from build123d import *

# Parameters (mm, degrees)
CROQUIS1_R              = 23.05
SALIENTE_EXTRUIR1_DEPTH = 25
CROQUIS2_R              = 19.05
CORTAR_EXTRUIR1_DEPTH   = 29
CROQUIS3_R              = 23.05
CROQUIS3_R_2            = 20.5
CORTAR_EXTRUIR2_DEPTH   = 5
CROQUIS4_R              = 30
SALIENTE_EXTRUIR3_DEPTH = 20
CROQUIS5_R              = 19.05
CORTAR_EXTRUIR3_DEPTH   = 20


with BuildPart() as part:
    # Croquis1 → Saliente-Extruir1 (new body)
    with BuildSketch(Plane.XY):
        Circle(CROQUIS1_R)
    extrude(amount=SALIENTE_EXTRUIR1_DEPTH)

    # Croquis2 → Cortar-Extruir1 (cut)
    with BuildSketch(Plane(origin=(0, 0, 0), x_dir=(-1, 0, 0), z_dir=(0, 0, -1))):
        Circle(CROQUIS2_R)
    extrude(amount=-CORTAR_EXTRUIR1_DEPTH, mode=Mode.SUBTRACT)

    # Croquis3 → Cortar-Extruir2 (cut)
    with BuildSketch(Plane(origin=(0, 0, 0), x_dir=(-1, 0, 0), z_dir=(0, 0, -1))):
        Circle(CROQUIS3_R)
        Circle(CROQUIS3_R_2, mode=Mode.SUBTRACT)
    extrude(amount=-CORTAR_EXTRUIR2_DEPTH, mode=Mode.SUBTRACT)

    # Croquis4 → Saliente-Extruir3 (add)
    with BuildSketch(Plane.XY.offset(25)):
        Circle(CROQUIS4_R)
    extrude(amount=-SALIENTE_EXTRUIR3_DEPTH)

    # Croquis5 → Cortar-Extruir3 (cut)
    with BuildSketch(Plane(origin=(0, 0, 5), x_dir=(-1, 0, 0), z_dir=(0, 0, -1))):
        Circle(CROQUIS5_R)
    extrude(amount=-CORTAR_EXTRUIR3_DEPTH, mode=Mode.SUBTRACT)


solid = part.part
Geometry check sheet. Reference: the model listing, model coordinates, mm. A direction names the side the tool comes from. Round coordinates to 2 decimals unless told otherwise and drop trailing zeros. Loops run counter-clockwise (first coordinate to the right, second up) from the corner with the lowest first, then second, coordinate; pieces in that order, holes last.
Item 1: Cross-section at D-D on x = 24. Record the boundary of the cut face in (y, z), then the cut area to 3 significant figures.
Item 2: Cross-section at C-C on z = 19.75. Record the boundary of the cut face in (x, y).
Item 3: Mould release check, pull along Y, two halves, no side actions. Record for faces 1 (the cylindrical face through (-29.97, 1.32, 15.14)), 2 (the cylindrical face through (15.12, -11.59, 12.32)), 3 (the flat face through (20, -6, 5)): pulls with the +Y half, pulls with the -Y half, needs draft (parallel to the pull), parting line crosses it, or undercut.
Item 4: Access from +Z, -Z, +X, -X, +Y, -Y to the whole of each face (thin tool, end or side, straight path). Record for faces 4 (the cylindrical face through (4.444, -20.013, 2.465)), 5 (the flat face through (14, -14, 0)).
Item 5: Thickness scan on line 1 (Y direction, x = 0, z = 16.25); line 2 (Z direction, x = 21.5, y = -14); line 3 (X direction, y = 10.5, z = 4.5). Record the ranges inside material, lowest first.
Item 6: Cross-section at A-A on y = 0. Record the boundary of the cut face in (x, z), then the cut area to 4 significant figures.
Item 7: Gauge pin test, flat ends, axial feed: pin 1 (10 mm diameter, centred on x = 8.5, z = 8, fed in from -Y); pin 2 (2 mm diameter, centred on y = -7, z = 13.5, fed in from -X); pin 3 (5 mm diameter, centred on y = -12, z = 6.5, fed in from -X); pin 4 (12 mm diameter, centred on x = 3.5, y = -19.5, fed in from -Z). Record the tip position at first contact, or that the pin passes through.
Answer sheet:
1. outline: (-18, 5) - (18, 5) - (18, 25) - (-18, 25) - close
1. area: 720 mm2
2. outline: circle Ø60 at (0, 0); hole circle Ø38.1 at (0, 0)
3. face 1: parting line crosses it
3. face 2: undercut
3. face 3: needs draft
4. face 4: -Z
4. face 5: -Z, +X, -X, +Y, -Y
5. line 1: y = -30 to -19.05, 19.05 to 30
5. line 2: z = 5 to 25
5. line 3: x = -17.61 to -15.9, 15.9 to 17.61
6. outline: (-30, 5) - (-20.5, 5) - (-20.5, 0) - (-19.05, 0) - (-19.05, 25) - (-30, 25) - close; (19.05, 0) - (20.5, 0) - (20.5, 5) - (30, 5) - (30, 25) - (19.05, 25) - close
6. area: 452.5 mm2
7. pin 1: stops at y = -29.8
7. pin 2: stops at x = -29.39
7. pin 3: stops at x = -28.46
7. pin 4: stops at z = 0
